Here's the drawing with two shaded views (mm, measured from the low corner). I have some questions. A direction names the side the tool comes from. Round coordinates to 2 decimals unless told otherwise and drop trailing zeros. Loops run counter-clockwise (first coordinate to the right, second up) from the corner with the lowest first, then second, coordinate; pieces in that order, holes last. Notation, with made-up numbers: M -30.5,-26 L 9.5,-26 A16 ccw 9.5,-7 Z; hole C 52,64.25 d8. An arc over 180 degrees is marked long. Answer as a JSON object with one key per item and string values.
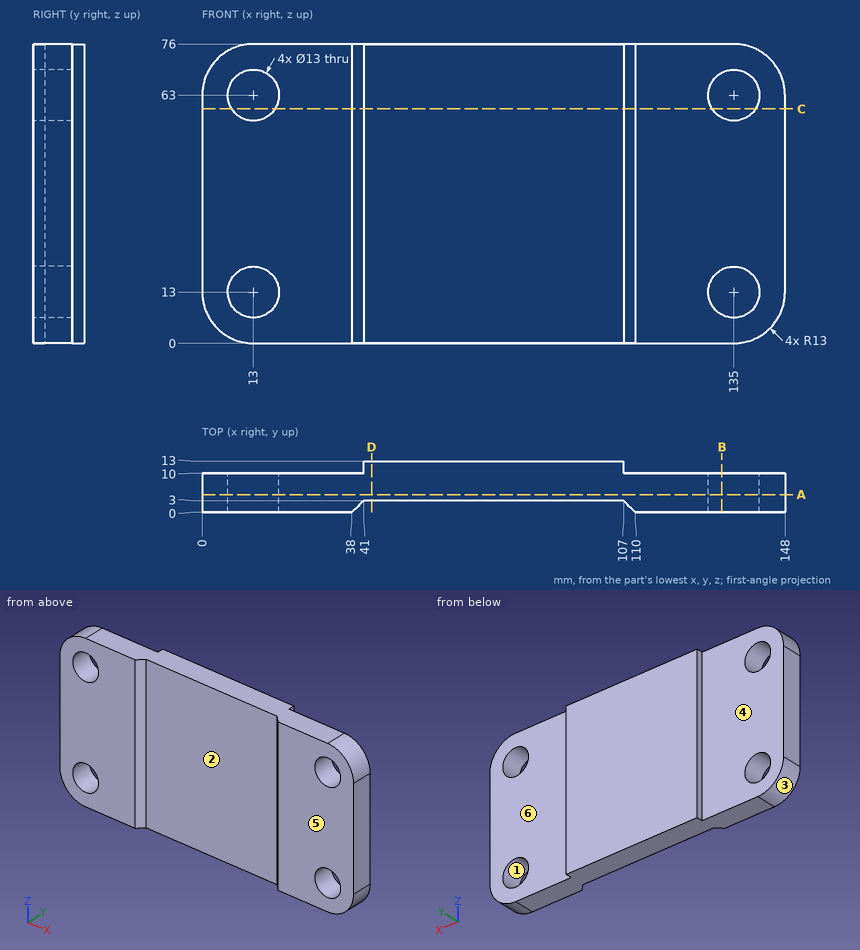
Item 1: I want a section at D-D on x = 43. List the corners of the cut face in (y, z) for me.
Solution:
{"outline": "M 3,0 L 13,0 L 13,76 L 3,76 Z"}
Item 2: I want a section at A-A on y = 4.5. List the corners of the cut face in (x, z) for me, plus the area to 3 significant figures.
Solution:
{"outline": "M 0,13 A13 ccw 13,0 L 135,0 A13 ccw 148,13 L 148,63 A13 ccw 135,76 L 13,76 A13 ccw 0,63 Z; hole C 13,13 d13; hole C 13,63 d13; hole C 135,13 d13; hole C 135,63 d13", "area": "10,600 mm2"}
Item 3: If I drill on L1, parallel to X at y = 9.25, z = 66.5; L2, parallel to Z at x = 7, y = 1.75; L3, parallel to Y at x = 29, z = 17.5, over which ranges is the centre line in solid material (lowest first)? Write a range as from..to.
Solution:
{"L1": "x = 0.48..7.52, 18.48..129.52, 140.48..147.52", "L2": "z = 1.47..10.5, 15.5..60.5, 65.5..74.53", "L3": "y = 0..10"}
Item 4: For P1, Ø0.9, axis at y = 11.5, z = 38.5, coming from the -X side; P2, Ø12.5, axis at x = 11, z = 32.5, coming from the +Y side; P3, Ø0.9, axis at y = 12, z = 39, coming from the +X side, each with a flat end and sliding along its axis, tell me the tip position at first contact or that it passes through.
Solution:
{"P1": "stops at x = 41", "P2": "stops at y = 10", "P3": "stops at x = 107"}
Item 5: I want a section at B-B on x = 132. List the corners of the cut face in (y, z) for me.
Solution:
{"outline": "M 0,0 L 10,0 L 10,7.23 L 0,7.23 Z; M 0,18.77 L 10,18.77 L 10,57.23 L 0,57.23 Z; M 0,68.77 L 10,68.77 L 10,76 L 0,76 Z"}
Item 6: For the marked faces 4, 5 and 6, which set-ups out of +Z, -Z, +X, -X, +Y, -Y let a thin tool reach every point of the face, with its end or its side?
Solution:
{"face 4": "+Z, -Z, -X, +Y", "face 5": "+Z, -Z, +X, -X, -Y", "face 6": "+Z, -Z, +X, +Y"}
Item 7: I want a section at C-C on z = 59.5. List the corners of the cut face in (x, y) for me, plus the area to 3 significant figures.
Solution:
{"outline": "M 0,0 L 7.52,0 L 7.52,10 L 0,10 Z; M 18.48,0 L 38,0 L 41,3 L 107,3 L 110,0 L 129.52,0 L 129.52,10 L 107,10 L 107,13 L 41,13 L 41,10 L 18.48,10 Z; M 140.48,0 L 148,0 L 148,10 L 140.48,10 Z", "area": "1,250 mm2"}
Item 8: We'd pull the mould along Z, two halves only. Please class the marked faces 1, 2 and 3: +Z half, -Z half, draft (parallel to the pull), parting line (faces both ways), or undercut.
Solution:
{"face 1": "undercut", "face 2": "draft", "face 3": "-Z half"}
